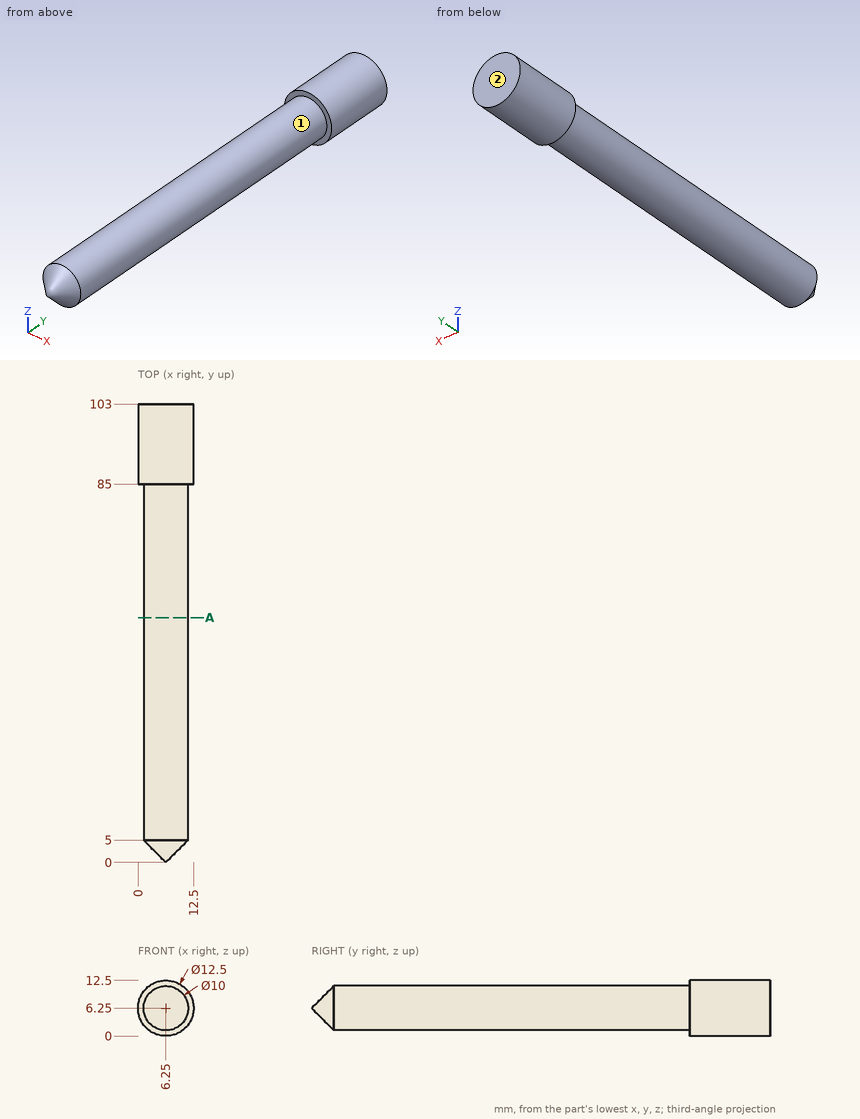
Here's the drawing with two shaded views (mm, measured from the low corner). I have some questions. A direction names the side the tool comes from. Give positions to 0.01 mm unless a question says otherwise; leave off trailing zeros. Loops run counter-clockwise (first coordinate to the right, second up) from the corner with the lowest first, then second, coordinate; pieces in that order, holes last. Notation, with made-up numbers: M -15,89.5 L 25,89.5 A17 cw 25,115.5 Z; hole C 59.5,83 d11. An arc over 180 degrees is marked long. Use one line per item in the form item = value. Start each with the question number.
(1) I want a section at A-A, the plane y = 55. Write out the boundary of the cut face in (x, z), and give its area (3 significant figures).
(2) Please list where these lines run through material, in increasing order: line 1 (X direction, y = 88.5, z = 6.75); line 2 (Y direction, x = 2.75, z = 1.5); line 3 (Z direction, x = 6.5, y = 8.5).
(3) On a 3-axis mill with a long thin cutter (end or side, diameter ignored), from which of +Z, -Z, +X, -X, +Y, -Y can I reach the whole of each face in a straight line? I mean the marked faces 1 and 2. Say none if no direction works.
(4) I'm going to push flat-ended pins straight in: P1, Ø6, axis at y = 32.5, z = 6.5, coming from the -X side; P2, Ø3, axis at x = 6.5, z = 10, coming from the -Y side. Where does each tip first touch, or does it pass through?
Worked out:
q1.outline = C 6.25,6.25 d10
q1.area = 78.5 mm²
q2.line_1 = 0.02 to 12.48
q2.line_2 = 85 to 103
q2.line_3 = 1.26 to 11.24
q3.face_1 = -Y
q3.face_2 = +Z, -Z, +X, -X, +Y
q4.P1 = 1.25
q4.P2 = 2.26
